from build123d import *

# Parameters (mm, degrees)
BOSS_EXTRUDE1_DEPTH              = 6.35
F_0_257_DIAMETER_HOLE1_D         = 6.5278
F_11_64_0_17188_DIAMETER_HOLE2_D = 4.365752
BOSS_EXTRUDE2_DEPTH              = 6.35
CHAMFER1_SIZE                    = 2
CHAMFER1_SIZE_2                  = 1.900651734
F_9_64_0_14063_DIAMETER_HOLE3_D  = 3.572002
CUT_EXTRUDE6_DEPTH               = 1.27
CUT_EXTRUDE6_DEPTH_BACK          = 3.175
SKETCH37_W                       = 6.696
SKETCH37_H                       = 6.696
FILLET2_R                        = 3.175


with BuildPart() as part:
    # Sketch1 → Boss-Extrude1 (new body)
    with BuildSketch(Plane.XY):
        with BuildLine():
            Line((3.956679664, 44.662837486), (6.340832795, 0.341085714))
            ThreePointArc((6.340832795, 0.341085714), (0, -6.35), (-6.340832795, 0.341085714))
            Line((-6.340832795, 0.341085714), (-3.956679664, 44.662837486))
            ThreePointArc((-3.956679664, 44.662837486), (0, 48.4124), (3.956679664, 44.662837486))
        make_face()
    extrude(amount=BOSS_EXTRUDE1_DEPTH)

    # F (0.257) Diameter Hole1 (through all)
    with Locations(Plane.XY.offset(6.35)):
        with Locations((0, 0)):
            Hole(F_0_257_DIAMETER_HOLE1_D / 2)

    # 11/64 (0.17188) Diameter Hole2 (through all)
    with Locations(Plane.XY.offset(6.35)):
        with Locations((0, 25.4)):
            Hole(F_11_64_0_17188_DIAMETER_HOLE2_D / 2)

    # Sketch8 → Boss-Extrude2 (add)
    with BuildSketch(Plane.XY.offset(6.35)):
        Polygon((4.48049686, 34.925), (3.956679664, 44.662837486), (3.751732363, 48.472837486), (-3.751732363, 48.472837486), (-3.956679664, 44.662837486), (-4.48049686, 34.925), (-4.72151149, 30.44450314), (0, 30.44450314), (4.72151149, 30.44450314), align=None)
    extrude(amount=BOSS_EXTRUDE2_DEPTH)

    # Chamfer1
    # the kernel refuses this chamfer: 2, 1.900651734 mm, written as the material it adds along each edge
    with BuildSketch(Plane(origin=(0, 44.45, 6.35), x_dir=(-0.31887891485273423, -0.9477954619338197, 0), z_dir=(0.9477954619338197, -0.31887891485273423, 0))) as chamfer1_piece_1_section:
        Polygon((3.9624, CHAMFER1_SIZE), (3.9624 + CHAMFER1_SIZE, 0), (3.9624, 0), align=None)
    chamfer1_piece_1 = revolve(axis=Axis((0, 44.45, 6.35), (0, 0, -1)), revolution_arc=322.809720089, mode=Mode.PRIVATE)
    chamfer1_piece_1 = split(chamfer1_piece_1, bisect_by=Plane(origin=(-3.847302471, 46.696175344, 4.621548789), z_dir=(0.9985563456862132, -0.05371428571428559, 0)), keep=Keep.TOP, mode=Mode.PRIVATE)
    chamfer1_piece_1 = split(chamfer1_piece_1, bisect_by=Plane(origin=(3.826743256, 47.078374128, 4.621548789), z_dir=(-0.9985563456862132, -0.05371428571428527, 0)), keep=Keep.TOP, mode=Mode.PRIVATE)
    chamfer1_piece_1 = split(chamfer1_piece_1, bisect_by=Plane(origin=(-3.562844962, 48.472837486, 4.621548789), z_dir=(0, -1, 0)), keep=Keep.TOP, mode=Mode.PRIVATE)
    add(chamfer1_piece_1)
    # the kernel refuses this chamfer: 2, 1.900651734 mm, written as the material it takes off along each edge
    with BuildSketch(Plane(origin=(-4.72151149, 30.44450314, 6.35), x_dir=(0.026237795181529237, 0.9996557297910176, 0), z_dir=(0, 0, 1))) as chamfer1_2_piece_1:
        Polygon((CHAMFER1_SIZE * 0.999621916911, -CHAMFER1_SIZE * 0.0274958766106), (CHAMFER1_SIZE_2 * 0.0262377951788, -CHAMFER1_SIZE_2 * 0.999655729687), (0, 0), align=None)
    extrude(amount=11.493365976, mode=Mode.SUBTRACT)
    with BuildSketch(Plane(origin=(4.72151149, 30.44450314, 6.35), x_dir=(-0.023285655605869076, 0.9997288523609813, 0), z_dir=(0, 0, 1))) as chamfer1_2_piece_2:
        Polygon((CHAMFER1_SIZE_2 * 0.999536361745, CHAMFER1_SIZE_2 * 0.0304476820407), (CHAMFER1_SIZE * 0.0232856556059, CHAMFER1_SIZE * 0.999728852361), (0, 0), align=None)
    extrude(amount=11.493365976, mode=Mode.SUBTRACT)

    # 9/64 (0.14063) Diameter Hole3 (through all)
    with Locations(Plane(origin=(6.340832795, 0.341085714, 0), x_dir=(0, 0, -1), z_dir=(0.9985563456862132, 0.05371428571428528, 0))):
        with Locations((-6.35, 38.676337841)):
            Hole(F_9_64_0_14063_DIAMETER_HOLE3_D / 2)

    # Sketch37 → Cut-Extrude6 (cut, two sides: drawn at the far end of the back side and taken through both)
    with BuildSketch(Plane(origin=(-1.14098275, -0.061375679, 0), x_dir=(0, 0, -1), z_dir=(0.9985563456862132, 0.05371428571428528, 0)).offset(-CUT_EXTRUDE6_DEPTH_BACK)):
        with Locations((-6.35, 38.676337841)):
            Rectangle(SKETCH37_W, SKETCH37_H)
    extrude(amount=CUT_EXTRUDE6_DEPTH + CUT_EXTRUDE6_DEPTH_BACK, mode=Mode.SUBTRACT)

    # Fillet2
    fillet2_edges = [part.edges().sort_by_distance(p)[0] for p in [
        (-3.751732363, 48.472837486, 9.294196206),
        (0, 48.472837486, 12.7),
    ]]
    fillet(fillet2_edges, radius=FILLET2_R)


solid = part.part
Design review of the part built by this model. Coordinates are the model's own, in mm. A direction names the side the tool comes from. Coordinates: 2 decimals unless noted, no trailing zeros. Order: outer loops, then holes, each group sorted by start corner. A loop starts at its lowest first (then second) coordinate and runs counter-clockwise, first axis right, second up. Notation, with made-up numbers: (83.5, 61) - (93.5, 61) arc R14 ccw to (93.5, 85) - close; hole circle Ø6 at (25, -36.5). An arc over 180 degrees is marked (long way). Put each result on its own line as item: value.
1) Take a section at D-D, the plane y = 33. Give the boundary of the cut face in (x, z).
Response values:
outline: (-4.58, 0) - (4.58, 0) - (4.58, 12.7) - (-4.58, 12.7) - close
2) Take a section at B-B, the plane z = 2.5. Give the boundary of the cut face in (x, y), and give its area (3 significant figures).
Response values:
outline: (-6.34, 0.34) arc R6.35 ccw (long way) to (6.34, 0.34) - (3.96, 44.66) arc R3.96 ccw to (-3.96, 44.66) - close; hole circle Ø6.53 at (0, 0); hole circle Ø4.37 at (0, 25.4)
area: 499 mm²
3) Tool access review of faces 4 (the face through (-3.73, 31.46, 9.48)), 5 (the face through (3.684, 31.407, 9.481)), 6 (the face through (-0.08, 48.41, 2.14)), 7 (the face through (-3.14, 35.21, 6.4)): name each direction out of +Z, -Z, +X, -X, +Y, -Y from which nothing blocks a thin tool from reaching the whole face with its end or side.
Response values:
face 4: +Z, -X, -Y
face 5: +Z, +X, -Y
face 6: -Z, +Y
face 7: -X
4) Take a section at C-C, the plane y = 25.4. Give the boundary of the cut face in (x, z).
Response values:
outline: (-4.99, 0) - (-2.18, 0) - (-2.18, 6.35) - (-4.99, 6.35) - close; (2.18, 0) - (4.99, 0) - (4.99, 6.35) - (2.18, 6.35) - close
5) The part is to be moulded in two halves that separate along Z. For faces 1 (the face through (0, 30.445, 9)), 2 (the face through (-3, 39, 9.698)), 3 (the face through (0.817, 47.567, 11.745)), say which applies: released by +Z, released by -Z, zero draft, split by the parting line, or undercut.
Response values:
face 1: zero draft
face 2: undercut
face 3: released by +Z
6) Wall thickness on L1, parallel to Y at x = 0, z = 4.5; L2, parallel to Y at x = 0, z = 1.75; L3, parallel to Y at x = 0, z = 5.25: over which ranges is each line inside the solid? List them lowest first. Write a range as from..to.
Response values:
L1: y = -6.35..-3.26, 3.26..23.22, 27.58..48.47
L2: y = -6.35..-3.26, 3.26..23.22, 27.58..48.41
L3: y = -6.35..-3.26, 3.26..23.22, 27.58..37.32, 40.14..48.47
7) Insertion check: P1, Ø4, axis at x = 0, y = 0, coming from the +Z side; P2, Ø1.7, axis at x = 1, z = 8.5, coming from the -Y side; P3, Ø5.5, axis at x = 0, y = 25.4, coming from the +Z side. Each pin has a flat end and moves straight along its axis. Give the tip position at first contact, or say it passes through.
Response values:
P1: passes through
P2: stops at y = 30.44
P3: stops at z = 6.35
